```python
from build123d import *

# Parameters (mm, degrees)
F0_R     = 2.15265
F1_DEPTH = 3.175
F2_R     = 6.34999


# Not quite as in the source:
# - a fillet or chamfer is up to 0.001 mm smaller than in the source, because OpenCascade refuses the exact size


with BuildPart() as f1:
    # F0 (on Top) → F1 (new body)
    with BuildSketch(Plane.XY):
        Polygon((12.7, 749.3), (0, 749.3), (0, 0), (-374.65, 0), (-374.65, -12.7), (387.35, -12.7), (387.35, 0), (12.7, 0), align=None)
        with Locations((-368.3, -6.35)):
            Circle(F0_R, mode=Mode.SUBTRACT)
        with Locations((6.35, -6.35)):
            Circle(F0_R, mode=Mode.SUBTRACT)
        with Locations((381, -6.35)):
            Circle(F0_R, mode=Mode.SUBTRACT)
        with Locations((6.35, 368.3)):
            Circle(F0_R, mode=Mode.SUBTRACT)
        with Locations((6.35, 742.95)):
            Circle(F0_R, mode=Mode.SUBTRACT)
    extrude(amount=F1_DEPTH)

    # F2 (radius 6.35 in the source; OpenCascade refuses exactly that, so slightly less here)
    f2_edges = [f1.edges().sort_by_distance(p)[0] for p in [
        (0, 749.3, 1.5875),
        (12.7, 749.3, 1.5875),
        (387.35, -12.7, 1.5875),
        (387.35, 0, 1.5875),
        (-374.65, -12.7, 1.5875),
        (-374.65, 0, 1.5875),
    ]]
    fillet(f2_edges, radius=F2_R)


solid = f1.part
```
Geometry check sheet. Reference: the model listing, model coordinates, mm. Coordinates: 2 decimals unless noted, no trailing zeros. Order: outer loops, then holes, each group sorted by start corner. A loop starts at its lowest first (then second) coordinate and runs counter-clockwise, first axis right, second up. Notation, with made-up numbers: (64, 41.25) - (102, 41.25) arc R19 ccw to (102, 57.25) - close; hole circle Ø9 at (78.5, 49.5). An arc over 180 degrees is marked (long way). Answer as a JSON object with one key per item and string values. Group by question number.
Item 1: Scan lines: probe 1 along X at (y, z) = (189.5, 1.95); probe 2 along Y at (x, z) = (129, 0.65). Record each from-to range of solid material in increasing order.
Item 2: Sectioned sample at C-C, the plane x = -306. Record the cut outline in (y, z) (3 decimals), and give its area (3 significant figures).
Item 3: Sectioned sample at A-A, the plane z = 2.4. Give the number of separate pieces and of enclosed holes in the cut face, and give its area (3 significant figures).
Item 4: Sectioned sample at B-B, the plane y = 482. Record the cut outline in (x, z) (3 decimals), and give its area (3 significant figures).
Item 5: Depth check by flat-ended pin: pin 1 Ø1 at (x, z) = (-248, 1) entering from +Y; pin 2 Ø2.5 at (x, y) = (6.35, 742.95) entering from -Z; pin 3 Ø1.6 at (y, z) = (316, 1.5) entering from -X. Enter the tip coordinate at first touch or a pass-through.
Resolved:
{
 "1": {"probe 1": "0 to 12.7", "probe 2": "-12.7 to 0"},
 "2": {"outline": "(-12.7, 0) - (0, 0) - (0, 3.175) - (-12.7, 3.175) - close", "area": "40.3 mm^2"},
 "3": {"separate pieces": "1", "enclosed holes": "5", "area": "19,100 mm^2"},
 "4": {"outline": "(0, 0) - (12.7, 0) - (12.7, 3.175) - (0, 3.175) - close", "area": "40.3 mm^2"},
 "5": {"pin 1": "y = 0", "pin 2": "through", "pin 3": "x = 0"}
}
